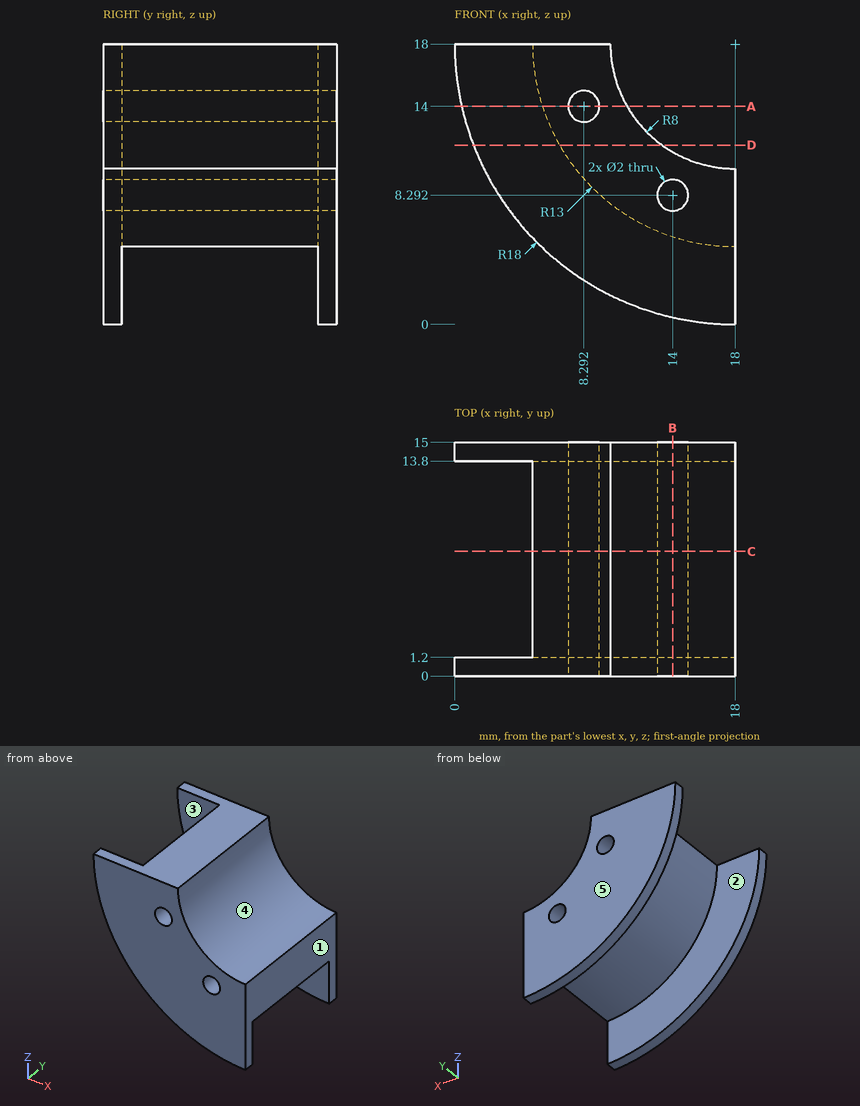
For this review, use the dimensioned drawing (mm, ordinates from the lowest corner) and the shaded views. A direction names the side the tool comes from. Coordinates: 2 decimals unless noted, no trailing zeros. Loops run counter-clockwise (first coordinate to the right, second up) from the corner with the lowest first, then second, coordinate; pieces in that order, holes last. Notation, with made-up numbers: (40.25, 50.25) -> (97.25, 50.25) arc R29 cw to (97.25, 86.25) -> close; hole circle Ø2 at (0, 13.25). An arc over 180 degrees is marked (long way). Write each question's results on one line, items separated by ' | '.
Q1. Machinability: for the marked faces 1 and 2, which of the approach directions +Z, -Z, +X, -X, +Y, -Y give a long, thin tool a straight path to every point of the face, cutting with its end or side? Answer none if there is none.
Taken from the geometry:
face 1: +Z, -Z, +X, +Y, -Y | face 2: -Z, -X
Q2. Add section D-D, the plane z = 11.5. State the section outline as (x, y) points (1 decimal).
Taken from the geometry:
outline: (1.2, 0) -> (13.3, 0) -> (13.3, 15) -> (1.2, 15) -> (1.2, 13.8) -> (6.7, 13.8) -> (6.7, 1.2) -> (1.2, 1.2) -> close
Q3. To check wall thickness, follow line 1 along Y through (x, z) = (12.25, 3.75); line 2 along Z through (x, y) = (8.5, 7) (1 decimal); line 3 along X through (y, z) = (6.5, 14.25). State the ranges of each line that lie inside material, in increasing order. Write a range as [from, to].
Taken from the geometry:
line 1: [0, 1.2], [13.8, 15] | line 2: [9.1, 13], [15, 18] | line 3: [5.55, 7.32], [9.26, 10.93]
Q4. Mouldability with a two-part tool opening along Y and no side actions: class the marked faces 3, 4 and 5 as +Y half, -Y half, draft (parallel to the pull), parting line (faces both ways), or undercut.
Taken from the geometry:
face 3: undercut | face 4: draft | face 5: +Y half
Q5. Add section C-C, the plane y = 8. State the section outline as (x, z) points, then the cut area to 3 significant figures.
Taken from the geometry:
outline: (5, 18) arc R13 ccw to (18, 5) -> (18, 10) arc R8 cw to (10, 18) -> close; hole circle Ø2 at (8.29, 14); hole circle Ø2 at (14, 8.29) | area: 76.2 mm²
Q6. Add section B-B, the plane x = 14. State the section outline as (y, z) points.
Taken from the geometry:
outline: (0, 0.45) -> (1.2, 0.45) -> (1.2, 5.63) -> (13.8, 5.63) -> (13.8, 0.45) -> (15, 0.45) -> (15, 7.29) -> (0, 7.29) -> close; (0, 9.29) -> (15, 9.29) -> (15, 11.07) -> (0, 11.07) -> close
Q7. For pin 1 Ø4 at (x, z) = (14.5, 11) entering from -Y; pin 2 Ø1 at (y, z) = (10.5, 13.5) entering from +X (1 decimal); pin 3 Ø4 at (y, z) = (3.5, 14) entering from -X (1 decimal), all flat-tipped, find the tip position at first contact; note any pin that passes through.
Taken from the geometry:
pin 1: y = 0 | pin 2: x = 11.8 | pin 3: x = 5.2
Q8. Add section A-A, the plane z = 14. State the section outline as (x, y) points.
Taken from the geometry:
outline: (0.45, 0) -> (7.29, 0) -> (7.29, 15) -> (0.45, 15) -> (0.45, 13.8) -> (5.63, 13.8) -> (5.63, 1.2) -> (0.45, 1.2) -> close; (9.29, 0) -> (11.07, 0) -> (11.07, 15) -> (9.29, 15) -> close
